```python
from build123d import *

# Parameters (mm, degrees)
SKETCH1_R                      = 6.15
BOSS_EXTRUDE1_DEPTH            = 13.5
F_2_7_2_7_DIAMETER_HOLE1_D     = 2.7
F_2_7_2_7_DIAMETER_HOLE1_DEPTH = 4
F_2_7_2_7_DIAMETER_HOLE1_TIP   = 0.811161836


with BuildPart() as part:
    # Sketch1 → Boss-Extrude1 (new body)
    with BuildSketch(Plane.XY):
        with BuildLine():
            Line((-9.5, 8), (-9.5, -8))
            Line((-9.5, -8), (0, -8))
            ThreePointArc((0, -8), (8, 0), (0, 8))
            Line((0, 8), (-9.5, 8))
        make_face()
        Circle(SKETCH1_R, mode=Mode.SUBTRACT)
    extrude(amount=BOSS_EXTRUDE1_DEPTH)

    # Ø2.7 (2.7) Diameter Hole1
    with Locations(Plane.ZY.offset(9.5)):
        with Locations((2.5, -5), (2.5, 5), (11, 5), (11, -5)):
            Hole(F_2_7_2_7_DIAMETER_HOLE1_D / 2, depth=F_2_7_2_7_DIAMETER_HOLE1_DEPTH)
            with Locations((0, 0, -(F_2_7_2_7_DIAMETER_HOLE1_DEPTH + F_2_7_2_7_DIAMETER_HOLE1_TIP / 2))):  # 118° drill point
                Cone(0, F_2_7_2_7_DIAMETER_HOLE1_D / 2, F_2_7_2_7_DIAMETER_HOLE1_TIP, mode=Mode.SUBTRACT)


solid = part.part
```
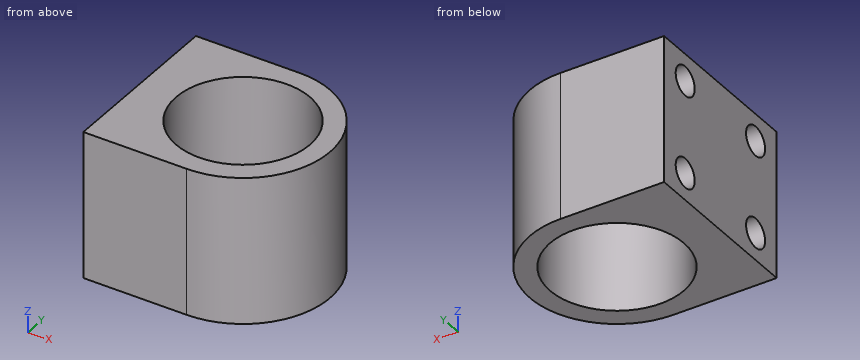
Could you check a few things on this model? Use its own coordinates, in mm. Round coordinates to 2 decimals unless told otherwise and drop trailing zeros. Loops run counter-clockwise (first coordinate to the right, second up) from the corner with the lowest first, then second, coordinate; pieces in that order, holes last.
Q1. I want a section at A-A (y = -3.25). Write out the boundary of the cut face in (x, z).
Q2. For P1, Ø6, axis at x = -2.5, y = 4.5, coming from the -Z side; P2, Ø1.6, axis at y = -5, z = 11, coming from the +X side; P3, Ø2, axis at y = -5, z = 2.5, coming from the +X side; P4, Ø2.5, axis at y = 5, z = 11, coming from the +X side, each with a flat end and sliding along its axis, tell me the tip position at first contact or that it passes through.
Q3. Please list where these lines run through material, in increasing order: L1, parallel to Z at x = -8.05, y = 5; L2, parallel to Y at x = -6.4, z = 11; L3, parallel to X at y = 1.25, z = 3.75.
Q4. I want a section at C-C (z = 7.75). Write out the boundary of the cut face in (x, y).
Q5. I want a section at B-B (x = -2.25). Write out the boundary of the cut face in (y, z).
Answer below:
1. outline: (-9.5, 0) - (-5.22, 0) - (-5.22, 13.5) - (-9.5, 13.5) - close; (5.22, 0) - (7.31, 0) - (7.31, 13.5) - (5.22, 13.5) - close
2. P1: stops at z = 0
2. P2: stops at x = 6.81
2. P3: stops at x = 6.93
2. P4: stops at x = 7.07
3. L1: z = 0 to 1.15, 3.85 to 9.65, 12.35 to 13.5
3. L2: y = -8 to -6.35, -3.65 to 3.65, 6.35 to 8
3. L3: x = -9.5 to -6.02, 6.02 to 7.9
4. outline: (-9.5, -8) - (0, -8) arc R8 ccw to (0, 8) - (-9.5, 8) - close; hole circle Ø12.3 at (0, 0)
5. outline: (-8, 0) - (-5.72, 0) - (-5.72, 13.5) - (-8, 13.5) - close; (5.72, 0) - (8, 0) - (8, 13.5) - (5.72, 13.5) - close
